The model under review builds one solid part; all positions refer to its coordinate system, in mm. Coordinates: 2 decimals unless noted, no trailing zeros. Write each loop counter-clockwise with the first axis right and the second up, starting at its lowest first coordinate (ties: lowest second). Pieces come first, ordered by that corner, then holes. Notation, with made-up numbers: (-3.75, 51) - (41.25, 51) arc R21 cw to (41.25, 79) - close; hole circle Ø1 at (3.5, 73.5). An arc over 180 degrees is marked (long way). Put each result on its own line as item: value. Start each with the question number.
Item 1: For pin 1 (1.6 mm diameter, centred on x = -201, y = 2, fed in from +Z); pin 2 (1 mm diameter, centred on y = 2, z = -5, fed in from +X), all flat-tipped, find the tip position at first contact; note any pin that passes through.
Item 2: Consider section A-A on x = 155. Give the boundary of the cut face in (y, z) (3 decimals).
Item 3: Consider section C-C on y = 1.7. Give the boundary of the cut face in (x, z), then the cut area to 3 significant figures.
Item 4: Consider section B-B on z = -28. Give the boundary of the cut face in (x, y) (3 decimals), then the cut area to 3 significant figures.
Item 5: To check wall thickness, follow L1, parallel to Z at x = -144, y = 2.1; L2, parallel to X at y = 1.5, z = 61; L3, parallel to X at y = 1.95, z = 8. State the ranges of each line that lie inside material, in increasing order. Write a range as [from, to].
```python
from build123d import *

# Parameters (mm, degrees)
SKETCH1_W           = 393.6492
SKETCH1_H           = 6.4008
SKETCH1_W_2         = 380.8984
SKETCH1_H_2         = 97.44075
BOSS_EXTRUDE1_DEPTH = 3.175


with BuildPart() as part:
    # Sketch1 → Boss-Extrude1 (new body)
    with BuildSketch(Plane(origin=(0, 0, 0), x_dir=(1, 0, 0), z_dir=(0, 1, 0))):
        Polygon((-203.2, 64.620775), (-203.2, -64.620775), (-196.85, -64.620775), (-196.85, -67.821175), (203.2, -67.821175), (203.2, -51.895375), (196.7992, -51.895375), (196.7992, 51.895375), (203.2, 51.895375), (203.2, 67.821175), (-196.85, 67.821175), (-196.85, 64.620775), align=None)
        with Locations((-0.0254, 58.270775)):
            Rectangle(SKETCH1_W, SKETCH1_H, mode=Mode.SUBTRACT)
        with Locations((-0.0254, -58.270775)):
            Rectangle(SKETCH1_W, SKETCH1_H, mode=Mode.SUBTRACT)
        Rectangle(SKETCH1_W_2, SKETCH1_H_2, mode=Mode.SUBTRACT)
    extrude(amount=BOSS_EXTRUDE1_DEPTH)


solid = part.part
```
Report:
1. pin 1: z = 64.62
1. pin 2: x = 196.8
2. outline: (0, -67.821) - (3.175, -67.821) - (3.175, -61.471) - (0, -61.471) - close; (0, -55.07) - (3.175, -55.07) - (3.175, -48.72) - (0, -48.72) - close; (0, 48.72) - (3.175, 48.72) - (3.175, 55.07) - (0, 55.07) - close; (0, 61.471) - (3.175, 61.471) - (3.175, 67.821) - (0, 67.821) - close
3. outline: (-203.2, -64.62) - (-196.85, -64.62) - (-196.85, -67.82) - (203.2, -67.82) - (203.2, -51.9) - (196.8, -51.9) - (196.8, 51.9) - (203.2, 51.9) - (203.2, 67.82) - (-196.85, 67.82) - (-196.85, 64.62) - (-203.2, 64.62) - close; hole (-196.85, -61.47) - (196.8, -61.47) - (196.8, -55.07) - (-196.85, -55.07) - close; hole (-196.85, 55.07) - (196.8, 55.07) - (196.8, 61.47) - (-196.85, 61.47) - close; hole (-190.45, -48.72) - (190.45, -48.72) - (190.45, 48.72) - (-190.45, 48.72) - close
3. area: 12,300 mm²
4. outline: (-203.2, 0) - (-190.449, 0) - (-190.449, 3.175) - (-203.2, 3.175) - close; (190.449, 0) - (196.799, 0) - (196.799, 3.175) - (190.449, 3.175) - close
4. area: 60.6 mm²
5. L1: [-67.82, -61.47], [-55.07, -48.72], [48.72, 55.07], [61.47, 67.82]
5. L2: [-203.2, -196.85], [196.8, 203.2]
5. L3: [-203.2, -190.45], [190.45, 196.8]
